from build123d import *

# Parameters (mm, degrees)
SKETCH025_W             = 107
SKETCH025_H             = 107
SKETCH025_W_2           = 82
SKETCH025_H_2           = 82
PAD005_DEPTH            = 1.75
SKETCH026_R             = 1.15
PAD006_DEPTH            = 1.75
FILLET008_R             = 3
FILLET009_R             = 2
CHAMFER014_SIZE2        = 2
CHAMFER014_SIZE         = 1.5
BODY005_PLACEMENT_ANGLE = 180


with BuildPart() as part:
    # Sketch025 → Pad005 (new body)
    with BuildSketch(Plane.XY):
        Rectangle(SKETCH025_W, SKETCH025_H)
        Rectangle(SKETCH025_W_2, SKETCH025_H_2, mode=Mode.SUBTRACT)
    extrude(amount=PAD005_DEPTH)

    # Sketch026 → Pad006 (join)
    with BuildSketch(Plane.XY):
        with BuildLine():
            ThreePointArc((-53.5, 38), (-61.5, 30), (-53.5, 22))
            Line((-53.5, 38), (-53.5, 22))
        make_face()
        with Locations((-57.25, 30)):
            Circle(SKETCH026_R, mode=Mode.SUBTRACT)
        with BuildLine():
            ThreePointArc((-53.5, -22), (-61.5, -30), (-53.5, -38))
            Line((-53.5, -22), (-53.5, -38))
        make_face()
        with Locations((-57.25, -30)):
            Circle(SKETCH026_R, mode=Mode.SUBTRACT)
        with BuildLine():
            Line((53.5, 38), (53.5, 22))
            ThreePointArc((53.5, 22), (61.5, 30), (53.5, 38))
        make_face()
        with Locations((57.25, 30)):
            Circle(SKETCH026_R, mode=Mode.SUBTRACT)
        with BuildLine():
            ThreePointArc((53.5, -38), (61.5, -30), (53.5, -22))
            Line((53.5, -22), (53.5, -38))
        make_face()
        with Locations((57.25, -30)):
            Circle(SKETCH026_R, mode=Mode.SUBTRACT)
    extrude(amount=PAD006_DEPTH)

    # Fillet008
    fillet008_edges = [part.edges().sort_by_distance(p)[0] for p in [
        (-53.5, 53.5, 0.875),
        (53.5, 53.5, 0.875),
        (53.5, -53.5, 0.875),
        (-53.5, -53.5, 0.875),
    ]]
    fillet(fillet008_edges, radius=FILLET008_R)

    # Fillet009
    fillet009_edges = [part.edges().sort_by_distance(p)[0] for p in [
        (-41, 41, 0.875),
        (41, 41, 0.875),
        (41, -41, 0.875),
        (-41, -41, 0.875),
    ]]
    fillet(fillet009_edges, radius=FILLET009_R)

    # Chamfer014
    chamfer014_edges = [part.edges().sort_by_distance(p)[0] for p in [
        (-41, 0, 1.75),
    ]]
    chamfer014_side = part.faces().sort_by_distance((-41, 0, 0.875))[0]
    chamfer(chamfer014_edges, length=CHAMFER014_SIZE, length2=CHAMFER014_SIZE2, reference=chamfer014_side)


with BuildPart() as part_1:
    # Body004 placement: moved
    add(part.part.moved(Location((0, 0, 21.5))))


with BuildPart() as part_2:
    # Body005 placement: moved
    add(part_1.part.rotate(Axis((0, 0, 0), (0, 1, 0)), BODY005_PLACEMENT_ANGLE))


solid = part_2.part
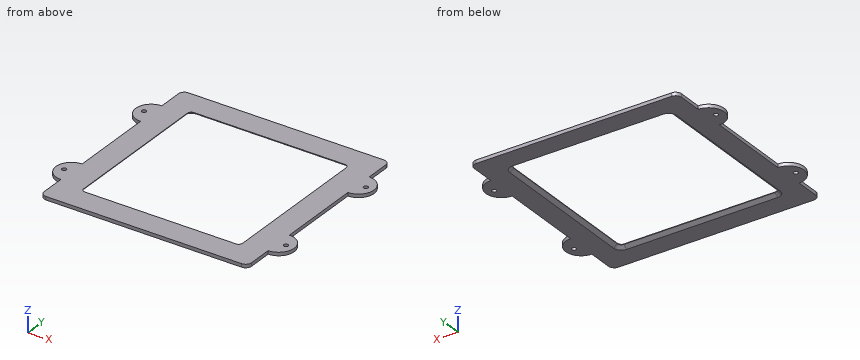
Input: part model. Units: mm. Frame: model coordinates. Give positions to 0.01 mm unless a question says otherwise; leave off trailing zeros. Loops run counter-clockwise (first coordinate to the right, second up) from the corner with the lowest first, then second, coordinate; pieces in that order, holes last. Notation, with made-up numbers: (50, 81) - (69, 81) arc R12 cw to (69, 102) - close; hole circle Ø9 at (-28, -5). An arc over 180 degrees is marked (long way). Use CSV: the item, a comma, the result in double quotes. Start each with the question number.
Item 1: Line query: line 1 (Y direction, x = -57.25, z = -21.85); line 2 (Y direction, x = -31, z = -21.7); line 3 (X direction, y = -33.5, z = -22.6). Output: solid intervals per line, ascending.
Item 2: Section C-C on z = -22.15. Return loops of the section in (x, y), then the cut area to 3 significant figures.
Item 3: Section A-A on y = -15. Return loops of the section in (x, z), then the cut area to 4 significant figures.
Item 4: Contact query for flat-ended pins moving along their axis: P1, Ø0.9, axis at y = -45.5, z = -22.5, coming from the -X side; P2, Ø0.5, axis at y = -42.5, z = -22.5, coming from the +X side. Output: stop coordinate, or through.
Ans:
1,line 1,"y = -37.07 to -31.15, -28.85 to -22.93, 22.93 to 28.85, 31.15 to 37.07"
1,line 2,"y = -53.5 to -41, 41 to 53.5"
1,line 3,"x = -60.69 to -42.13, 42.13 to 60.69"
2,outline,"(-53.5, -50.5) arc R3 ccw to (-50.5, -53.5) - (50.5, -53.5) arc R3 ccw to (53.5, -50.5) - (53.5, -38) arc R8 ccw to (53.5, -22) - (53.5, 22) arc R8 ccw to (53.5, 38) - (53.5, 50.5) arc R3 ccw to (50.5, 53.5) - (-50.5, 53.5) arc R3 ccw to (-53.5, 50.5) - (-53.5, 38) arc R8 ccw to (-53.5, 22) - (-53.5, -22) arc R8 ccw to (-53.5, -38) - close; hole circle Ø2.3 at (-57.25, -30); hole circle Ø2.3 at (-57.25, 30); hole (-41.53, -39) arc R2.53 ccw to (-39, -41.53) - (39, -41.53) arc R2.53 ccw to (41.53, -39) - (41.53, 39) arc R2.53 ccw to (39, 41.53) - (-39, 41.53) arc R2.53 ccw to (-41.53, 39) - close; hole circle Ø2.3 at (57.25, -30); hole circle Ø2.3 at (57.25, 30)"
2,area,"4,930 mm2"
3,outline,"(-53.5, -23.25) - (-43, -23.25) - (-41, -21.75) - (-41, -21.5) - (-53.5, -21.5) - close; (41, -21.75) - (43, -23.25) - (53.5, -23.25) - (53.5, -21.5) - (41, -21.5) - close"
3,area,"40.75 mm2"
4,P1,"stops at x = -53.5"
4,P2,"stops at x = 53.5"
